Geometry: final body of the model. Coordinates: model frame, mm. Round coordinates to 2 decimals unless told otherwise and drop trailing zeros. Order: outer loops, then holes, each group sorted by start corner. A loop starts at its lowest first (then second) coordinate and runs counter-clockwise, first axis right, second up. Notation, with made-up numbers: (-5, 35) - (0, 35) arc R21 cw to (0, 66) - close; hole circle Ø1 at (79.25, 68.5). An arc over 180 degrees is marked (long way). Put each result on its own line as item: value. Start each with the question number.
(1) Section A-A (y = 0). Output: boundary loops of the cut face in (x, z).
(2) Pin query (flat end, axial travel): P1, Ø6, axis at y = -3.5, z = 95.5, coming from the -X side; P2, Ø3.5, axis at x = 2, y = 0, coming from the +Z side; P3, Ø1, axis at x = 1.5, z = 241.5, coming from the +Y side. Return the tip coordinate at first contact, or that it passes through.
(3) Section C-C (z = 462.5). Output: boundary loops of the cut face in (x, y).
(4) Material intervals for L1, parallel to Y at x = 0, z = 239.25; L2, parallel to Y at x = 0, z = 639; L3, parallel to Y at x = 0, z = 140.5, sorted ascending. Write a range as [from, to].
from build123d import *

# Parameters (mm, degrees)
SKETCH1_R           = 4.699
SKETCH1_R_2         = 3.75
BOSS_EXTRUDE1_DEPTH = 215.9
SKETCH6_R           = 7.62
SKETCH6_R_2         = 5.5
BOSS_EXTRUDE2_DEPTH = 671.6


with BuildPart() as part:
    # Sketch1 → Boss-Extrude1 (new body)
    with BuildSketch(Plane.XY):
        Circle(SKETCH1_R)
        Circle(SKETCH1_R_2, mode=Mode.SUBTRACT)
    extrude(amount=BOSS_EXTRUDE1_DEPTH)

    # Sketch5 → Revolve1 (revolve)
    with BuildSketch(Plane(origin=(0, 0, 0), x_dir=(1, 0, 0), z_dir=(0, 1, 0))):
        Polygon((-4.699, -208.123650762), (-7.62, -236.448520775), (-5.08, -236.448520775), (-5.08, -245.9), (-3.58, -245.9), (-3.58, -215.9), (-4.699, -215.9), align=None)
    revolve(axis=Axis((0, 0, 215.9), (0, 0, 1)))

    # Sketch6 → Boss-Extrude2 (add)
    with BuildSketch(Plane.XY.offset(236.448520775)):
        Circle(SKETCH6_R)
        Circle(SKETCH6_R_2, mode=Mode.SUBTRACT)
    extrude(amount=BOSS_EXTRUDE2_DEPTH)


solid = part.part
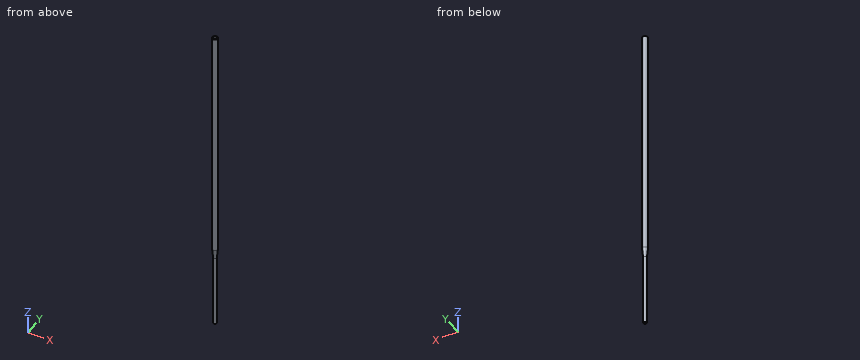
Checks:
1. outline: (-7.62, 236.45) - (-4.7, 208.12) - (-4.7, 0) - (-3.75, 0) - (-3.75, 215.9) - (-3.58, 215.9) - (-3.58, 245.9) - (-5.08, 245.9) - (-5.08, 236.45) - (-5.5, 236.45) - (-5.5, 908.05) - (-7.62, 908.05) - close; (3.58, 215.9) - (3.75, 215.9) - (3.75, 0) - (4.7, 0) - (4.7, 208.12) - (7.62, 236.45) - (7.62, 908.05) - (5.5, 908.05) - (5.5, 236.45) - (5.08, 236.45) - (5.08, 245.9) - (3.58, 245.9) - close
2. P1: stops at x = -4.67
2. P2: stops at z = 245.9
2. P3: stops at y = 7.55
3. outline: circle Ø15.24 at (0, 0); hole circle Ø11 at (0, 0)
4. L1: y = [-7.62, -5.5], [-5.08, -3.58], [3.58, 5.08], [5.5, 7.62]
4. L2: y = [-7.62, -5.5], [5.5, 7.62]
4. L3: y = [-4.7, -3.75], [3.75, 4.7]
